For this review, take the finished solid that the model builds, in its own axes (mm). A direction names the side the tool comes from. Coordinates: 2 decimals unless noted, no trailing zeros. Loops run counter-clockwise (first coordinate to the right, second up) from the corner with the lowest first, then second, coordinate; pieces in that order, holes last. Notation, with made-up numbers: (85, 23) - (137, 23) arc R22 ccw to (137, 45) - close; hole circle Ø10 at (34.25, 56.25). An arc over 180 degrees is marked (long way). Use one line per item in the form item = value. Start each with the question number.
1. Draft analysis for pull direction Y (two halves, no side actions). For faces 4 (the face through (-79.1, -2, -1)), 5 (the face through (-1, 6.35, -1)), 6 (the face through (-30.26, -5.04, -44.35)), 7 (the face through (-6, -11.08, 44)), state which applies: +Y half, -Y half, draft (parallel to the pull), parting line (faces both ways), or undercut.
2. Add section A-A on x = 40. Give the boundary of the cut face in (y, z) (3 decimals), and give its area (3 significant figures).
3. Add section B-B on z = 23.5. Give the boundary of the cut face in (x, y).
4. Add section C-C on x = -50. Give the boundary of the cut face in (y, z), and give its area (3 significant figures).
5. For pin 1 Ø1 at (x, z) = (-7.5, 26) entering from -Y; pin 2 Ø2.5 at (y, z) = (-5.54, -45.93) entering from -X; pin 3 Ø0.8 at (x, y) = (27.5, -2) entering from -Z, all flat-tipped, find the tip position at first contact; note any pin that passes through.
6. To check wall thickness, follow probe 1 along Z at (x, y) = (-32, -5.25); probe 2 along X at (y, z) = (-1.25, -13.5); probe 3 along Y at (x, z) = (-22.5, -32). State the ranges of each line that lie inside material, in increasing order.
7. Machinability: for faces 1 (the face through (12.446, -3.7, -46)), 2 (the face through (-76, -3, -49.1)), 3 (the face through (75.881, -9.631, -47.572)), which of the approach directions +Z, -Z, +X, -X, +Y, -Y give a long, thin tool a straight path to every point of the face, cutting with its end or side? Answer none if there is none.
```python
from build123d import *

# Parameters (mm, degrees)
IZIM1_W                     = 158.200000084
IZIM1_H                     = 98.199999942
Y_KSEKLIK_EKSTR_ZYON1_DEPTH = 6.35
Y_KSEKLIK_EKSTR_ZYON2_DEPTH = 34.142000042
Y_KSEKLIK_EKSTR_ZYON3_DEPTH = 34.650000042
IZIM5_R                     = 1.651
KES_EKSTR_ZYON1_DEPTH       = 38.1
IZIM6_R                     = 1.651
KES_EKSTR_ZYON2_DEPTH       = 34.142000042
IZIM7_W                     = 98.200002037
IZIM7_H                     = 11.08
Y_KSEKLIK_EKSTR_ZYON4_DEPTH = 6.35
IZIM10_W                    = 98.200002037
IZIM10_H                    = 11.08
Y_KSEKLIK_EKSTR_ZYON5_DEPTH = 6.35
IZIM12_W                    = 145.500000084
IZIM12_H                    = 11.08
Y_KSEKLIK_EKSTR_ZYON6_DEPTH = 6.35
RADYUS1_R                   = 5.08
RADYUS2_R                   = 5.08
IZIM15_R                    = 1.651
KES_EKSTR_ZYON3_DEPTH       = 6.35


with BuildPart() as part:
    # Çizim1 → Yükseklik-Ekstrüzyon1 (new body)
    with BuildSketch(Plane(origin=(0, 0, 0), x_dir=(1, 0, 0), z_dir=(0, 1, 0))):
        Rectangle(IZIM1_W, IZIM1_H)
    extrude(amount=Y_KSEKLIK_EKSTR_ZYON1_DEPTH)

    # Çizim2 → Yükseklik-Ekstrüzyon2 (add)
    with BuildSketch(Plane(origin=(-47.096000042, 0, 0), x_dir=(0, 0, -1), z_dir=(1, 0, 0))):
        with BuildLine():
            Line((49.100004162, 4.89e-07), (42.750004162, 4.89e-07))
            Line((42.750004162, 4.89e-07), (42.750004162, -2.799659899))
            ThreePointArc((42.750004162, -2.799659899), (45.925004162, -9.728237327), (49.100004162, -2.799659899))
            Line((49.100004162, -2.799659899), (49.100004162, 4.89e-07))
        make_face()
    extrude(amount=Y_KSEKLIK_EKSTR_ZYON2_DEPTH)


with BuildPart() as y_kseklik_ekstr_zyon3_tool:
    # Çizim3 → Yükseklik-Ekstrüzyon3 (new body)
    with BuildSketch(Plane.ZY.offset(-47.096000042)):
        with BuildLine():
            Line((-42.749997505, -7.075e-06), (-49.099997505, -7.075e-06))
            Line((-49.099997505, -7.075e-06), (-49.099997505, -2.799667463))
            ThreePointArc((-49.099997505, -2.799667463), (-45.924997505, -9.728244892), (-42.749997505, -2.799667463))
            Line((-42.749997505, -2.799667463), (-42.749997505, -7.075e-06))
        make_face()
    extrude(amount=Y_KSEKLIK_EKSTR_ZYON3_DEPTH)


with BuildPart() as part_1:
    add(part.part)


with BuildPart() as part_2:
    # Yükseklik-Ekstrüzyon3: joined with y_kseklik_ekstr_zyon3_tool
    add(part_1.part.fuse(y_kseklik_ekstr_zyon3_tool.part, tol=0.00001))

    # Çizim5 → Kes-Ekstrüzyon1 (cut)
    with BuildSketch(Plane(origin=(47.096000042, 0, 0), x_dir=(0, 0, -1), z_dir=(1, 0, 0))):
        with Locations((45.924997505, -5.536489024)):
            Circle(IZIM5_R)
    extrude(amount=-KES_EKSTR_ZYON1_DEPTH, mode=Mode.SUBTRACT)

    # Çizim6 → Kes-Ekstrüzyon2 (cut)
    with BuildSketch(Plane.ZY.offset(47.096000042)):
        with Locations((-45.925004162, -5.536481459)):
            Circle(IZIM6_R)
    extrude(amount=-KES_EKSTR_ZYON2_DEPTH, mode=Mode.SUBTRACT)

    # Çizim7 → Yükseklik-Ekstrüzyon4 (add)
    with BuildSketch(Plane.ZY.offset(79.100000042)):
        with Locations((-1.047e-06, -5.54)):
            Rectangle(IZIM7_W, IZIM7_H)
    extrude(amount=-Y_KSEKLIK_EKSTR_ZYON4_DEPTH)

    # Çizim10 → Yükseklik-Ekstrüzyon5 (add)
    with BuildSketch(Plane(origin=(79.100000042, 0, 0), x_dir=(0, 0, -1), z_dir=(1, 0, 0))):
        with Locations((1.047e-06, -5.54)):
            Rectangle(IZIM10_W, IZIM10_H)
    extrude(amount=-Y_KSEKLIK_EKSTR_ZYON5_DEPTH)

    # Çizim12 → Yükseklik-Ekstrüzyon6 (add)
    with BuildSketch(Plane.XY.offset(49.099999971)):
        with Locations((0, -5.54)):
            Rectangle(IZIM12_W, IZIM12_H)
    extrude(amount=-Y_KSEKLIK_EKSTR_ZYON6_DEPTH)

    # Radyus1
    radyus1_edges = [part_2.edges().sort_by_distance(p)[0] for p in [
        (75.925000042, -11.08, -49.100002066),
    ]]
    fillet(radyus1_edges, radius=RADYUS1_R)

    # Radyus2
    radyus2_edges = [part_2.edges().sort_by_distance(p)[0] for p in [
        (-75.925000042, -11.08, -49.100002066),
    ]]
    fillet(radyus2_edges, radius=RADYUS2_R)

    # Çizim15 → Kes-Ekstrüzyon3 (cut)
    with BuildSketch(Plane.ZY.offset(79.100000042)):
        with Locations((-45.925004162, -5.536481459)):
            Circle(IZIM15_R)
    extrude(amount=-KES_EKSTR_ZYON3_DEPTH, mode=Mode.SUBTRACT)


solid = part_2.part
```
Conclusion:
q1.face_4 = draft
q1.face_5 = +Y half
q1.face_6 = undercut
q1.face_7 = -Y half
q2.outline = (-11.08, 42.75) - (0, 42.75) - (0, -42.75) - (-2.8, -42.75) arc R4.192 ccw (long way) to (-2.8, -49.1) - (6.35, -49.1) - (6.35, 49.1) - (-11.08, 49.1) - close; hole circle Ø3.302 at (-5.536, -45.925)
q2.area = 752 mm^2
q3.outline = (-79.1, -11.08) - (-72.75, -11.08) - (-72.75, 0) - (72.75, 0) - (72.75, -11.08) - (79.1, -11.08) - (79.1, 6.35) - (-79.1, 6.35) - close
q4.outline = (-11.08, 42.75) - (0, 42.75) - (0, -49.1) - (6.35, -49.1) - (6.35, 49.1) - (-11.08, 49.1) - close
q4.area = 694 mm^2
q5.pin_1 = 0
q5.pin_2 = 72.75
q5.pin_3 = -49.1
q6.probe_1 = -50.11 to -47.55, -44.3 to -41.74, 42.75 to 49.1
q6.probe_2 = -79.1 to -72.75, 72.75 to 79.1
q6.probe_3 = 0 to 6.35
q7.face_1 = -Z, -Y
q7.face_2 = -Z, -X, +Y, -Y
q7.face_3 = -Z, +X, -Y
